from build123d import *

# Parameters (mm, degrees)
SKETCH1_W                       = 38
SKETCH1_H                       = 10.2
MAIN_BASE_DEPTH                 = 46.5
SKETCH2_R                       = 28.7
FREE_SPACE_DEPTH                = 6
BRACKETS1_START                 = 21.51023
BRACKETS1_DEPTH                 = 24.98977
BRACKETS2_START                 = -46.5
BRACKETS2_DEPTH                 = 24.98977
BRACKET_HOLES_DEPTH             = 54.040173454
BRACKET_HOLES_DEPTH_BACK        = 54.040173454
SKETCH5_W                       = 3.5
SKETCH5_H                       = 16.989769876
BOLT_HOLES_DEPTH                = 54.040173454
BOLT_HOLES_DEPTH_BACK           = 54.040173454
SKETCH6_R                       = 2.25
NUT_START                       = 5.1
NUT_SLOTS_DEPTH                 = 4.5
SKETCH8_W                       = 38
SKETCH8_H                       = 18
MOTOR_BASE_DEPTH                = 36.5
MOTOR_START                     = 19
SKETCH9_R                       = 1.1
MOTOR_BRACKETS1_DEPTH           = 2.95
MOTOR_START_2                   = -16.05
SKETCH9_2_R                     = 1.1
MOTOR_BRACKETS2_DEPTH           = 2.95
SKETCH10_R                      = 1.05
MOTOR_DRIVER_MOUNT_HOLES1_DEPTH = 10


with BuildPart() as part:
    # Sketch1 → Main_base (new, symmetric)
    with BuildSketch(Plane.XY):
        Rectangle(SKETCH1_W, SKETCH1_H)
    extrude(amount=MAIN_BASE_DEPTH, both=True)

    # Sketch2 → Free space (cut)
    with BuildSketch(Plane.XZ.offset(5.1)):
        Circle(SKETCH2_R)
    extrude(amount=-FREE_SPACE_DEPTH, mode=Mode.SUBTRACT)

    # Sketch3 → Brackets1 (add)
    with BuildSketch(Plane.XY.offset(BRACKETS1_START)):
        Polygon((25, 1.6), (25, -1.6), (19, -5.1), (19, 5.1), align=None)
        Polygon((-25, 1.6), (-19, 5.1), (-19, -5.1), (-25, -1.6), align=None)
    extrude(amount=BRACKETS1_DEPTH)

    # Sketch3<2> → Brackets2 (add)
    with BuildSketch(Plane.XY.offset(BRACKETS2_START)):
        Polygon((25, 1.6), (25, -1.6), (19, -5.1), (19, 5.1), align=None)
        Polygon((-25, 1.6), (-19, 5.1), (-19, -5.1), (-25, -1.6), align=None)
    extrude(amount=BRACKETS2_DEPTH)

    # Sketch5 → Bracket holes (cut, two sides: drawn at the far end of the back side and taken through both)
    with BuildSketch(Plane(origin=(0, 0, 0), x_dir=(1, 0, 0), z_dir=(0, 1, 0)).offset(-BRACKET_HOLES_DEPTH_BACK)):
        with Locations((20.75, -34.005115062)):
            Rectangle(SKETCH5_W, SKETCH5_H)
        with Locations((-20.75, -34.005115062)):
            Rectangle(SKETCH5_W, SKETCH5_H)
        with Locations((-20.75, 34.005115062)):
            Rectangle(SKETCH5_W, SKETCH5_H)
        with Locations((20.75, 34.005115062)):
            Rectangle(SKETCH5_W, SKETCH5_H)
    extrude(amount=BRACKET_HOLES_DEPTH + BRACKET_HOLES_DEPTH_BACK, mode=Mode.SUBTRACT)

    # Sketch6 → Bolt holes (cut, two sides: drawn at the far end of the back side and taken through both)
    with BuildSketch(Plane(origin=(0, 0, 0), x_dir=(1, 0, 0), z_dir=(0, 1, 0)).offset(-BOLT_HOLES_DEPTH_BACK)):
        with Locations(Location((-13, 39.5, 0), (0, 0, 270))):
            Circle(SKETCH6_R)
        with Locations(Location((-13, -39.5, 0), (0, 0, 270))):
            Circle(SKETCH6_R)
        with Locations(Location((13, -39.5, 0), (0, 0, 270))):
            Circle(SKETCH6_R)
        with Locations(Location((13, 39.5, 0), (0, 0, 270))):
            Circle(SKETCH6_R)
    extrude(amount=BOLT_HOLES_DEPTH + BOLT_HOLES_DEPTH_BACK, mode=Mode.SUBTRACT)

    # Sketch7 → Nut slots (cut)
    with BuildSketch(Plane(origin=(0, 0, 0), x_dir=(1, 0, 0), z_dir=(0, 1, 0)).offset(NUT_START)):
        Polygon((13, 35.256475), (16.675000452, 37.3782375), (16.675000452, 41.6217625), (13, 43.743525), (9.324999548, 41.6217625), (9.324999548, 37.3782375), align=None)
        Polygon((-9.324999548, 37.3782375), (-13, 35.256475), (-16.675000452, 37.3782375), (-16.675000452, 41.6217625), (-13, 43.743525), (-9.324999548, 41.6217625), align=None)
        Polygon((-13, -35.256475), (-16.675000452, -37.3782375), (-16.675000452, -41.6217625), (-13, -43.743525), (-9.324999548, -41.6217625), (-9.324999548, -37.3782375), align=None)
        Polygon((9.324999548, -37.3782375), (13, -35.256475), (16.675000452, -37.3782375), (16.675000452, -41.6217625), (13, -43.743525), (9.324999548, -41.6217625), align=None)
    extrude(amount=-NUT_SLOTS_DEPTH, mode=Mode.SUBTRACT)

    # Sketch8 → Motor base (add)
    with BuildSketch(Plane(origin=(0, 5.1, 0), x_dir=(1, 0, 0), z_dir=(0, 1, 0))):
        Rectangle(SKETCH8_W, SKETCH8_H)
    extrude(amount=MOTOR_BASE_DEPTH)

    # Sketch9 → Motor brackets1 (add)
    # profile 1 of 4: a face of its own
    with BuildSketch(Plane(origin=(0, 0, 0), x_dir=(0, 0, -1), z_dir=(1, 0, 0)).offset(MOTOR_START)):
        Polygon((-9, 41.6), (-11.5, 41.6), (-14.5, 38.6), (-14.5, 19.6), (-11.5, 16.6), (-9, 16.6), align=None)
        with Locations((-12, 21.1)):
            Circle(SKETCH9_R, mode=Mode.SUBTRACT)
        with Locations((-12, 37.1)):
            Circle(SKETCH9_R, mode=Mode.SUBTRACT)
    # profile 2 of 4: a face of its own
    with BuildSketch(Plane(origin=(0, 0, 0), x_dir=(0, 0, -1), z_dir=(1, 0, 0)).offset(MOTOR_START)):
        Polygon((-37.5, 5.1), (-12.5, 5.1), (-12.5, 7.6), (-15.5, 10.6), (-34.5, 10.6), (-37.5, 7.6), align=None)
        with Locations((-33, 8.1)):
            Circle(SKETCH9_R, mode=Mode.SUBTRACT)
        with Locations((-17, 8.1)):
            Circle(SKETCH9_R, mode=Mode.SUBTRACT)
    # profile 3 of 4: a face of its own
    with BuildSketch(Plane(origin=(0, 0, 0), x_dir=(0, 0, -1), z_dir=(1, 0, 0)).offset(MOTOR_START)):
        Polygon((11.5, 41.6), (14.5, 38.6), (14.5, 19.6), (11.5, 16.6), (9, 16.6), (9, 41.6), align=None)
        with Locations((12, 37.1)):
            Circle(SKETCH9_R, mode=Mode.SUBTRACT)
        with Locations((12, 21.1)):
            Circle(SKETCH9_R, mode=Mode.SUBTRACT)
    # profile 4 of 4: a face of its own
    with BuildSketch(Plane(origin=(0, 0, 0), x_dir=(0, 0, -1), z_dir=(1, 0, 0)).offset(MOTOR_START)):
        Polygon((15.5, 10.6), (12.5, 7.6), (12.5, 5.1), (37.5, 5.1), (37.5, 7.6), (34.5, 10.6), align=None)
        with Locations((17, 8.1)):
            Circle(SKETCH9_R, mode=Mode.SUBTRACT)
        with Locations((33, 8.1)):
            Circle(SKETCH9_R, mode=Mode.SUBTRACT)
    extrude(amount=-MOTOR_BRACKETS1_DEPTH)

    # Sketch9<2> → Motor brackets2 (add)
    # profile 1 of 4: a face of its own
    with BuildSketch(Plane(origin=(0, 0, 0), x_dir=(0, 0, -1), z_dir=(1, 0, 0)).offset(MOTOR_START_2)):
        Polygon((-9, 41.6), (-11.5, 41.6), (-14.5, 38.6), (-14.5, 19.6), (-11.5, 16.6), (-9, 16.6), align=None)
        with Locations((-12, 21.1)):
            Circle(SKETCH9_2_R, mode=Mode.SUBTRACT)
        with Locations((-12, 37.1)):
            Circle(SKETCH9_2_R, mode=Mode.SUBTRACT)
    # profile 2 of 4: a face of its own
    with BuildSketch(Plane(origin=(0, 0, 0), x_dir=(0, 0, -1), z_dir=(1, 0, 0)).offset(MOTOR_START_2)):
        Polygon((-37.5, 5.1), (-12.5, 5.1), (-12.5, 7.6), (-15.5, 10.6), (-34.5, 10.6), (-37.5, 7.6), align=None)
        with Locations((-33, 8.1)):
            Circle(SKETCH9_2_R, mode=Mode.SUBTRACT)
        with Locations((-17, 8.1)):
            Circle(SKETCH9_2_R, mode=Mode.SUBTRACT)
    # profile 3 of 4: a face of its own
    with BuildSketch(Plane(origin=(0, 0, 0), x_dir=(0, 0, -1), z_dir=(1, 0, 0)).offset(MOTOR_START_2)):
        Polygon((11.5, 41.6), (14.5, 38.6), (14.5, 19.6), (11.5, 16.6), (9, 16.6), (9, 41.6), align=None)
        with Locations((12, 37.1)):
            Circle(SKETCH9_2_R, mode=Mode.SUBTRACT)
        with Locations((12, 21.1)):
            Circle(SKETCH9_2_R, mode=Mode.SUBTRACT)
    # profile 4 of 4: a face of its own
    with BuildSketch(Plane(origin=(0, 0, 0), x_dir=(0, 0, -1), z_dir=(1, 0, 0)).offset(MOTOR_START_2)):
        Polygon((15.5, 10.6), (12.5, 7.6), (12.5, 5.1), (37.5, 5.1), (37.5, 7.6), (34.5, 10.6), align=None)
        with Locations((17, 8.1)):
            Circle(SKETCH9_2_R, mode=Mode.SUBTRACT)
        with Locations((33, 8.1)):
            Circle(SKETCH9_2_R, mode=Mode.SUBTRACT)
    extrude(amount=-MOTOR_BRACKETS2_DEPTH)

    # Sketch10 → motor_driver_mount_holes1 (cut)
    with BuildSketch(Plane.ZY.offset(19)):
        with Locations((-5.5, 14.9)):
            Circle(SKETCH10_R)
        with Locations((-5.5, 7.9)):
            Circle(SKETCH10_R)
        with Locations(Location((5.5, 7.9, 0), (0, 0, 180))):
            Circle(SKETCH10_R)
        with Locations(Location((5.5, 14.9, 0), (0, 0, 180))):
            Circle(SKETCH10_R)
    motor_driver_mount_holes1 = extrude(amount=-MOTOR_DRIVER_MOUNT_HOLES1_DEPTH, mode=Mode.SUBTRACT)

    # motor_driver_mount_holes2: motor_driver_mount_holes1 across plane
    add(motor_driver_mount_holes1.mirror(Plane(origin=(0, 0, 0), x_dir=(0, 0, 1), z_dir=(1, 0, 0))), mode=Mode.SUBTRACT)


solid = part.part
Geometry check sheet. Reference: the model listing, model coordinates, mm. A direction names the side the tool comes from. Give positions to 0.01 mm unless a question says otherwise; leave off trailing zeros. Order: outer loops, then holes, each group sorted by start corner. A loop starts at its lowest first (then second) coordinate and runs counter-clockwise, first axis right, second up. Notation, with made-up numbers: M -3.5,42 L 24.5,42 A14 ccw 24.5,52 Z; hole C -13.75,82 d10. An arc over 180 degrees is marked long. Use a Markdown table: item, result.
Item 1: Depth check by flat-ended pin: P1, Ø3.5, axis at y = 37.1, z = 12, coming from the -X side; P2, Ø1.2, axis at x = -17.5, z = -11, coming from the -Y side; P3, Ø6, axis at x = -13.5, z = -38, coming from the +Y side. Enter the tip coordinate at first touch or a pass-through.
Answers follow:
| item | result |
|---|---|
| P1 | stops at x = -19 |
| P2 | stops at y = 0.9 |
| P3 | stops at y = 8.68 |
Item 2: Section check B-B (z = -33). Record the cut outline in (x, y), and give its area (3 significant figures).
Answers follow:
| item | result |
|---|---|
| outline | M -25,-1.6 L -22.5,-3.06 L -22.5,3.06 L -25,1.6 Z; M -19,-5.1 L 19,-5.1 L 19,7 L 16.05,7 L 16.05,5.1 L -16.05,5.1 L -16.05,7 L -19,7 Z; M -19,9.2 L -16.05,9.2 L -16.05,10.6 L -19,10.6 Z; M 16.05,9.2 L 19,9.2 L 19,10.6 L 16.05,10.6 Z; M 22.5,-3.06 L 25,-1.6 L 25,1.6 L 22.5,3.06 Z |
| area | 430 mm2 |
Item 3: Section check D-D (y = 29.5). Record the cut outline in (x, z), and give its area (3 significant figures).
Answers follow:
| item | result |
|---|---|
| outline | M -19,-14.5 L -16.05,-14.5 L -16.05,-9 L 16.05,-9 L 16.05,-14.5 L 19,-14.5 L 19,14.5 L 16.05,14.5 L 16.05,9 L -16.05,9 L -16.05,14.5 L -19,14.5 Z |
| area | 749 mm2 |
Item 4: Draft check along Y on faces 6 (the flat face through (0, -5.1, -37)), 7 (the flat face through (17.5, 9.1, -36)), 8 (the cylindrical face through (13.099, -2.29, -41.748)), 9 (the flat face through (9, 15, -6)). Enter one of: +Y half, -Y half, draft (parallel to the pull), parting line (faces both ways), or undercut.
Answers follow:
| item | result |
|---|---|
| face 6 | -Y half |
| face 7 | +Y half |
| face 8 | draft |
| face 9 | undercut |
Item 5: Material ranges on line 1 along X through (y, z) = (-1.5, -37); line 2 along X through (y, z) = (-3.25, 39.5); line 3 along Z through (x, y) = (13, -1), recorded low to high.
Answers follow:
| item | result |
|---|---|
| line 1 | x = -25 to -22.5, -19 to 19, 22.5 to 25 |
| line 2 | x = -19 to -15.25, -10.75 to 10.75, 15.25 to 19 |
| line 3 | z = -46.5 to -41.75, -37.25 to -25.59, 25.59 to 37.25, 41.75 to 46.5 |
Item 6: Section check A-A (y = 37.1). Record the cut outline in (x, z), and give its area (3 significant figures).
Answers follow:
| item | result |
|---|---|
| outline | M -19,-14.5 L -16.05,-14.5 L -16.05,-13.1 L -19,-13.1 Z; M -19,-10.9 L -16.05,-10.9 L -16.05,-9 L 16.05,-9 L 16.05,-10.9 L 19,-10.9 L 19,10.9 L 16.05,10.9 L 16.05,9 L -16.05,9 L -16.05,10.9 L -19,10.9 Z; M -19,13.1 L -16.05,13.1 L -16.05,14.5 L -19,14.5 Z; M 16.05,-14.5 L 19,-14.5 L 19,-13.1 L 16.05,-13.1 Z; M 16.05,13.1 L 19,13.1 L 19,14.5 L 16.05,14.5 Z |
| area | 723 mm2 |
Item 7: Section check C-C (z = 17). Record the cut outline in (x, y), and give its area (3 significant figures).
Answers follow:
| item | result |
|---|---|
| outline | M -19,0.9 L 19,0.9 L 19,7 L 16.05,7 L 16.05,5.1 L -16.05,5.1 L -16.05,7 L -19,7 Z; M -19,9.2 L -16.05,9.2 L -16.05,10.6 L -19,10.6 Z; M 16.05,9.2 L 19,9.2 L 19,10.6 L 16.05,10.6 Z |
| area | 179 mm2 |
Item 8: Tool access check on faces 1 (the flat face through (16.05, 8, 25)), 2 (the flat face through (-17.5, 18.1, -13)), 3 (the flat face through (22.5, 0, -34)), 4 (the flat face through (11.19, 2.88, 42.7)), 5 (the flat face through (18, 6, 37.5)). Record the directions out of +Z, -Z, +X, -X, +Y, -Y that give a thin tool (end or side, any length) a straight path to the whole face; none if there is none.
Answers follow:
| item | result |
|---|---|
| face 1 | +Z, +Y |
| face 2 | -Z, +X, -X |
| face 3 | +Y, -Y |
| face 4 | +Y |
| face 5 | +Z, +X, -X, +Y |
